from build123d import *

# Parameters (mm, degrees)
SKETCH1_R           = 2.5
BOSS_EXTRUDE1_DEPTH = 190
SKETCH2_W           = 136.127535613
SKETCH2_H           = 180
CUT_EXTRUDE2_DEPTH  = 58
SKETCH3_W           = 45
SKETCH3_H           = 180
CUT_EXTRUDE3_DEPTH  = 3
BOSS_EXTRUDE2_START = 180
BOSS_EXTRUDE2_DEPTH = 180
SKETCH7_W           = 180
SKETCH7_H           = 22.5
CUT_EXTRUDE13_DEPTH = 30
SKETCH9_W           = 7.5
SKETCH9_H           = 22
CUT_EXTRUDE14_DEPTH = 3
BOSS_EXTRUDE3_DEPTH = 180


with BuildPart() as part:
    # Sketch1 → Boss-Extrude1 (new body)
    with BuildSketch(Plane.XY):
        with BuildLine():
            Line((0, 0), (47, 0))
            Line((47, 0), (37, 4.663076582))
            ThreePointArc((37, 4.663076582), (33.312668804, 10.778986497), (37.584760477, 16.501747909))
            Line((37.584760477, 16.501747909), (55, 16.501747909))
            ThreePointArc((55, 16.501747909), (62.367611495, 22.598786451), (57.756393324, 30.976867682))
            ThreePointArc((57.756393324, 30.976867682), (12.567155409, 46.120826206), (-33.970281413, 56.400596496))
            ThreePointArc((-33.970281413, 56.400596496), (-42.672566196, 49.617635726), (-35.197896825, 41.501747909))
            Line((-35.197896825, 41.501747909), (-20, 41.501747909))
            ThreePointArc((-20, 41.501747909), (-12.928932188, 38.572815721), (-10, 31.501747909))
            Line((-10, 31.501747909), (-10, 10))
            ThreePointArc((-10, 10), (-7.071067812, 2.928932188), (0, 0))
        make_face()
        with Locations((55, 24.001747909)):
            Circle(SKETCH1_R, mode=Mode.SUBTRACT)
        with Locations((-35.197896825, 49.001747909)):
            Circle(SKETCH1_R, mode=Mode.SUBTRACT)
    extrude(amount=BOSS_EXTRUDE1_DEPTH)

    # Sketch2 → Cut-Extrude2 (cut)
    with BuildSketch(Plane(origin=(0, 62.46968133, 0), x_dir=(1, 0, 0), z_dir=(0, 1, 0))):
        with Locations((11.703146866, -95)):
            Rectangle(SKETCH2_W, SKETCH2_H)
    extrude(amount=-CUT_EXTRUDE2_DEPTH, mode=Mode.SUBTRACT)

    # Sketch3 → Cut-Extrude3 (cut)
    with BuildSketch(Plane(origin=(0, 4.46968133, 0), x_dir=(1, 0, 0), z_dir=(0, 1, 0))):
        with Locations((14.168398989, -95)):
            Rectangle(SKETCH3_W, SKETCH3_H)
    extrude(amount=-CUT_EXTRUDE3_DEPTH, mode=Mode.SUBTRACT)



with BuildPart() as body_2:
    # Sketch4 → Boss-Extrude2 (new body)
    with BuildSketch(Plane(origin=(0, 0, 185), x_dir=(-1, 0, 0), z_dir=(0, 0, -1)).offset(BOSS_EXTRUDE2_START)):
        with BuildLine():
            Line((-30, 26.46968133), (-30, 1.46968133))
            Line((-30, 1.46968133), (5.218588256, 1.46968133))
            ThreePointArc((5.218588256, 1.46968133), (8.723126806, 5.110515495), (10, 10))
            Line((10, 10), (10, 26.46968133))
            Line((10, 26.46968133), (-30, 26.46968133))
        make_face()
        with BuildLine():
            Line((-27.5, 23.96968133), (7.5, 23.96968133))
            Line((7.5, 23.96968133), (7.5, 10))
            ThreePointArc((7.5, 10), (6.696815143, 6.62321648), (4.459288815, 3.96968133))
            Line((4.459288815, 3.96968133), (-27.5, 3.96968133))
            Line((-27.5, 3.96968133), (-27.5, 23.96968133))
        make_face(mode=Mode.SUBTRACT)
    extrude(amount=-BOSS_EXTRUDE2_DEPTH)

    # Sketch7 → Cut-Extrude13 (cut)
    with BuildSketch(Plane(origin=(30, 0, 0), x_dir=(0, 0, -1), z_dir=(1, 0, 0))):
        with Locations((-95, 12.71968133)):
            Rectangle(SKETCH7_W, SKETCH7_H)
    extrude(amount=-CUT_EXTRUDE13_DEPTH, mode=Mode.SUBTRACT)

    # Sketch9 → Cut-Extrude14 (cut)
    with BuildSketch(Plane(origin=(0, 26.46968133, 0), x_dir=(1, 0, 0), z_dir=(0, 1, 0))):
        with Locations((26.25, -46)):
            Rectangle(SKETCH9_W, SKETCH9_H)
    cut_extrude14 = extrude(amount=-CUT_EXTRUDE14_DEPTH, mode=Mode.SUBTRACT)

    # Mirror1: Cut-Extrude14 across plane
    add(cut_extrude14.mirror(Plane.XY.offset(95)), mode=Mode.SUBTRACT)


with BuildPart() as part_1:
    add(part.part)

    add(body_2.part)  # Boss-Extrude3 merges body 2
    # Sketch10 → Boss-Extrude3 (add)
    with BuildSketch(Plane(origin=(0, 0, 185), x_dir=(-1, 0, 0), z_dir=(0, 0, -1))):
        Polygon((-36.668398989, 1.46968133), (-36.668398989, 4.46968133), (0, 1.46968133), align=None)
    extrude(amount=BOSS_EXTRUDE3_DEPTH)


solid = part_1.part
Here's how the part is built. I have some questions about the finished solid (model axes, mm). A direction names the side the tool comes from. Give positions to 0.01 mm unless a question says otherwise; leave off trailing zeros. Order: outer loops, then holes, each group sorted by start corner. A loop starts at its lowest first (then second) coordinate and runs counter-clockwise, first axis right, second up. Notation, with made-up numbers: M -35.75,49 L -28.75,49 A21 cw -28.75,65 Z; hole C -13,-11 d1. An arc over 180 degrees is marked long. Answer as a JSON object with one key per item and string values. Group by question number.
1) I'm going to push flat-ended pins straight in: pin 1 Ø8 at (x, y) = (55, 24) entering from +Z; pin 2 Ø0.8 at (y, z) = (25, 143) entering from +X; pin 3 Ø2.5 at (x, z) = (50.5, 187.5) entering from -Y; pin 4 Ø1.5 at (x, z) = (-28.5, 186.5) entering from -Y. Where does each tip first touch, or does it pass through?
2) Suppose I cut it at A-A, the plane z = 54. Write out the boundary of the cut face in (x, y).
3) Suppose I cut it at D-D, the plane y = 37.5. Write out the boundary of the cut face in (x, z).
4) On a 3-axis mill with a long thin cutter (end or side, diameter ignored), from which of +Z, -Z, +X, -X, +Y, -Y can I reach the whole of each face in a straight line? I mean faces 4 (the flat face through (-28, 41.502, 187)), 5 (the flat face through (12, 23.97, 96)), 6 (the flat face through (10, 26.47, 94)). Say none if no direction works.
5) We'd pull the mould along Z, two halves only. Please class faces 1 (the flat face through (-10, 19, 94)), 2 (the flat face through (9, 29, 0)), 3 (the flat face through (-7.5, 17, 94)): pulls with the +Z half, pulls with the -Z half, needs draft (parallel to the pull), parting line crosses it, or undercut.
6) Suppose I cut it at C-C, the plane x = 18. Write out the boundary of the cut face in (y, z), plus the area to 3 significant figures.
7) Please list where these lines run through material, in increasing order: L1, parallel to Z at x = 50.5, y = 31.5; L2, parallel to X at y = 24.5, z = 119.5; L3, parallel to Y at x = 55, z = 188. Write a range as [from, to].
8) Suppose I cut it at B-B, the plane x = 40.5. Write out the boundary of the cut face in (y, z).
Results found:
{
 "1": {"pin 1": "z = 190", "pin 2": "x = 22.5", "pin 3": "y = 16.5", "pin 4": "y = 41.5"},
 "2": {"outline": "M -10,10 A10 ccw 0,0 L 47,0 L 37.41,4.47 L 36.67,4.47 L 0,1.47 L 0,3.97 L -4.46,3.97 A7.5 cw -7.5,10 L -7.5,23.97 L 22.5,23.97 L 22.5,26.47 L -10,26.47 Z"},
 "3": {"outline": "M -12,0 L 40.19,0 L 40.19,5 L -12,5 Z; M -12,185 L 40.19,185 L 40.19,190 L -12,190 Z"},
 "4": {"face 4": "+Z, -Z, -X, -Y", "face 5": "+X", "face 6": "+X, -X, +Y"},
 "5": {"face 1": "needs draft", "face 2": "pulls with the -Z half", "face 3": "undercut"},
 "6": {"outline": "M 0,0 L 44.58,0 L 44.58,5 L 26.47,5 L 26.47,185 L 44.58,185 L 44.58,190 L 0,190 Z; hole M 2.94,5 L 23.97,5 L 23.97,185 L 2.94,185 Z", "area": "1,430 mm²"},
 "7": {"L1": "[0, 5], [185, 190]", "L2": "[-10, 30]", "L3": "[16.5, 21.5], [26.5, 32.06]"},
 "8": {"outline": "M 0,0 L 3.03,0 L 3.03,190 L 0,190 Z; M 16.5,0 L 37.39,0 L 37.39,5 L 16.5,5 Z; M 16.5,185 L 37.39,185 L 37.39,190 L 16.5,190 Z"}
}
